from build123d import *

# Parameters (mm, degrees)
SKETCH_1_W      = 43
SKETCH_1_H      = 35
EXTRUDE_1_DEPTH = 140
SKETCH_2_R      = 2.5
EXTRUDE_2_DEPTH = 15
FILLET_1_R      = 3


with BuildPart() as part:
    # Эскиз1 → Бобышка-Вытянуть1 (new body)
    with BuildSketch(Plane.XY):
        Rectangle(SKETCH_1_W, SKETCH_1_H)
    extrude(amount=EXTRUDE_1_DEPTH)

    # Эскиз2 → Бобышка-Вытянуть2 (add)
    with BuildSketch(Plane.XY.offset(140)):
        with Locations((15.734743007, 3.598639962)):
            Circle(SKETCH_2_R)
        with Locations((15.734743007, -4.492095401)):
            Circle(SKETCH_2_R)
    extrude(amount=EXTRUDE_2_DEPTH)

    # Скругление1
    fillet_1_edges = [part.edges().sort_by_distance(p)[0] for p in [
        (-21.5, 0, 140),
        (0, -17.5, 140),
        (21.5, 0, 140),
        (0, -17.5, 0),
        (-21.5, 0, 0),
        (0, 17.5, 0),
        (21.5, 0, 0),
        (0, 17.5, 140),
        (21.5, -17.5, 70),
        (-21.5, -17.5, 70),
        (-21.5, 17.5, 70),
        (21.5, 17.5, 70),
    ]]
    fillet(fillet_1_edges, radius=FILLET_1_R)


solid = part.part
Read the model definition and answer for the solid it produces. Units are mm, in the model's axes. Give positions to 0.01 mm unless a question says otherwise; leave off trailing zeros. Write each loop counter-clockwise with the first axis right and the second up, starting at its lowest first coordinate (ties: lowest second). Pieces come first, ordered by that corner, then holes. Notation, with made-up numbers: (-35.75, 26.5) - (12.25, 26.5) arc R6 ccw to (12.25, 34.5) - close; hole circle Ø11 at (53.5, -30.75). An arc over 180 degrees is marked (long way). Return JSON: item names as keys, results as strings.
Q1. Consider line 1 along Z through (x, y) = (18, -1.5); line 2 along Y through (x, z) = (-9.5, 138); line 3 along Y through (x, z) = (-19, 64.5). Determine where each line is inside the solid, lowest interval first. Write a range as [from, to].
Reply:
{"line 1": "[0, 140]", "line 2": "[-17.33, 17.33]", "line 3": "[-17.46, 17.46]"}
Q2. A cutting plane is placed at A-A, the plane y = -0.5. Determine the outline of the cut face in (x, z), and give its area (3 significant figures).
Reply:
{"outline": "(-21.5, 3) arc R3 ccw to (-18.5, 0) - (18.5, 0) arc R3 ccw to (21.5, 3) - (21.5, 137) arc R3 ccw to (18.5, 140) - (-18.5, 140) arc R3 ccw to (-21.5, 137) - close", "area": "6,010 mm²"}
Q3. A cutting plane is placed at B-B, the plane x = 3.5. Determine the outline of the cut face in (y, z).
Reply:
{"outline": "(-17.5, 3) arc R3 ccw to (-14.5, 0) - (14.5, 0) arc R3 ccw to (17.5, 3) - (17.5, 137) arc R3 ccw to (14.5, 140) - (-14.5, 140) arc R3 ccw to (-17.5, 137) - close"}
Q4. Given P1, Ø2, axis at x = -14.5, y = 0, coming from the +Z side, flat-ended and moving along its own axis, determine where the tip first touches the part or whether it passes through.
Reply:
{"P1": "z = 140"}
Q5. For a pull along Y with two mould halves and no side action, classify faces 1 (the face through (13.75, -6.01, 147.4)), 2 (the face through (20.6, 0.2, 139.14)), 3 (the face through (0.26, -16.64, 0.9)), 4 (the face through (0.26, 16.64, 0.9)) as released by +Y, released by -Y, zero draft, split by the parting line, or undercut.
Reply:
{"face 1": "undercut", "face 2": "zero draft", "face 3": "released by -Y", "face 4": "released by +Y"}
